Answer from the drawing. Dimensions are ordinates in mm from the lowest x, y and z of the part. A direction names the side the tool comes from. Round coordinates to 2 decimals unless told otherwise and drop trailing zeros. Loops run counter-clockwise (first coordinate to the right, second up) from the corner with the lowest first, then second, coordinate; pieces in that order, holes last. Notation, with made-up numbers: (-38.5, 75.5) - (-19.5, 75.5) arc R12 cw to (-19.5, 85.5) - close; hole circle Ø7 at (64, 43). An arc over 180 degrees is marked (long way). Answer as CSV lines item,"result".
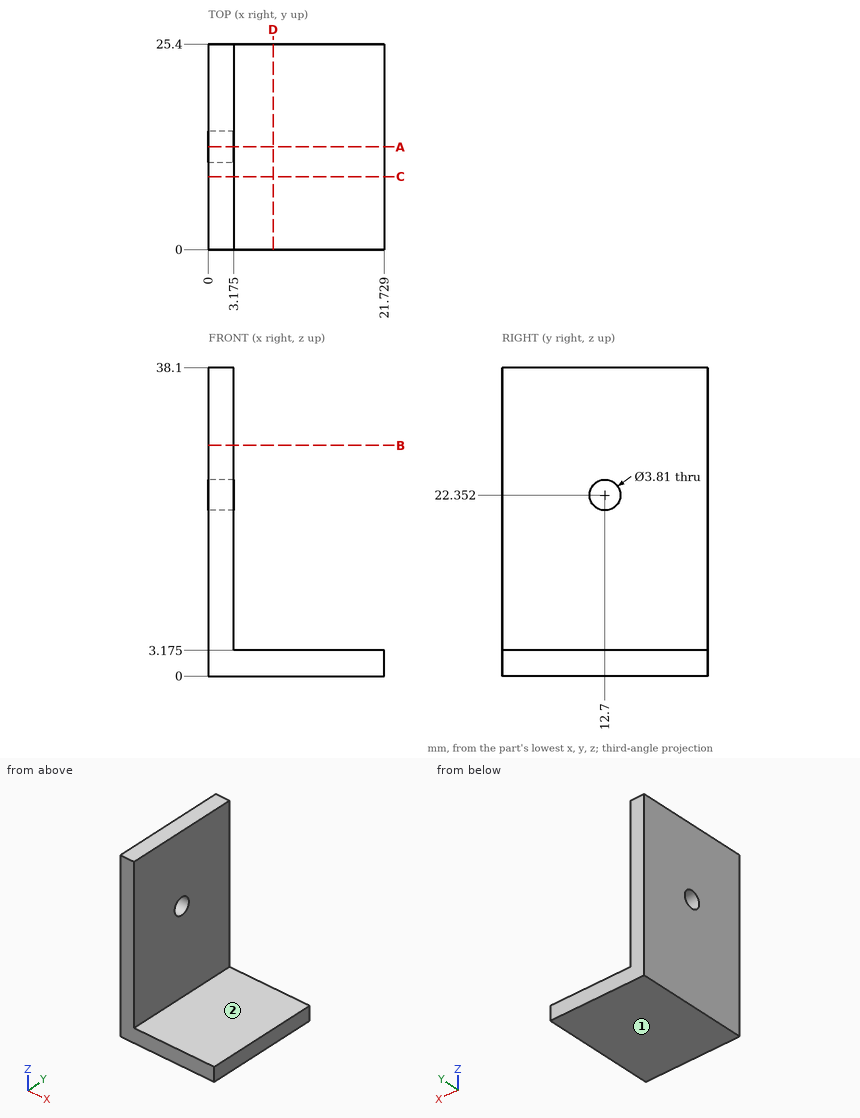
1) Find the intervals of material crossed by line 1 (Z direction, x = 1.3, y = 12.7); line 2 (X direction, y = 3.25, z = 35) (3 decimals), in increasing order.
Entries:
line 1,"z = 0 to 20.45, 24.26 to 38.1"
line 2,"x = 0 to 3.175"
2) Each of these flat-tipped pins is pushed along its axis until it touches: P1, Ø12, axis at x = 18.5, y = 18, coming from the +Z side (3 decimals); P2, Ø12.5, axis at y = 13, z = 21, coming from the +X side (3 decimals). Where does it stop, or does it pass through?
Entries:
P1,"stops at z = 3.175"
P2,"stops at x = 3.175"
3) A cutting plane is placed at B-B, the plane z = 28.5. Determine the outline of the cut face in (x, y) (3 decimals).
Entries:
outline,"(0, 0) - (3.175, 0) - (3.175, 25.4) - (0, 25.4) - close"
4) A tool of negligible diameter and unlimited length cuts with its end or side. For the marked faces 1 and 2, from which of +Z, -Z, +X, -X, +Y, -Y can it reach the whole face along a straight path? Write none if from no direction.
Entries:
face 1,"-Z, +X, -X, +Y, -Y"
face 2,"+Z, +X, +Y, -Y"
5) A cutting plane is placed at D-D, the plane x = 8. Determine the outline of the cut face in (y, z) (3 decimals), plus the area to 3 significant figures.
Entries:
outline,"(0, 0) - (25.4, 0) - (25.4, 3.175) - (0, 3.175) - close"
area,"80.6 mm^2"
6) A cutting plane is placed at C-C, the plane y = 9. Determine the outline of the cut face in (x, z) (3 decimals).
Entries:
outline,"(0, 0) - (21.729, 0) - (21.729, 3.175) - (3.175, 3.175) - (3.175, 38.1) - (0, 38.1) - close"
7) A cutting plane is placed at A-A, the plane y = 12.7. Determine the outline of the cut face in (x, z) (3 decimals).
Entries:
outline,"(0, 0) - (21.729, 0) - (21.729, 3.175) - (3.175, 3.175) - (3.175, 20.447) - (0, 20.447) - close; (0, 24.257) - (3.175, 24.257) - (3.175, 38.1) - (0, 38.1) - close"
